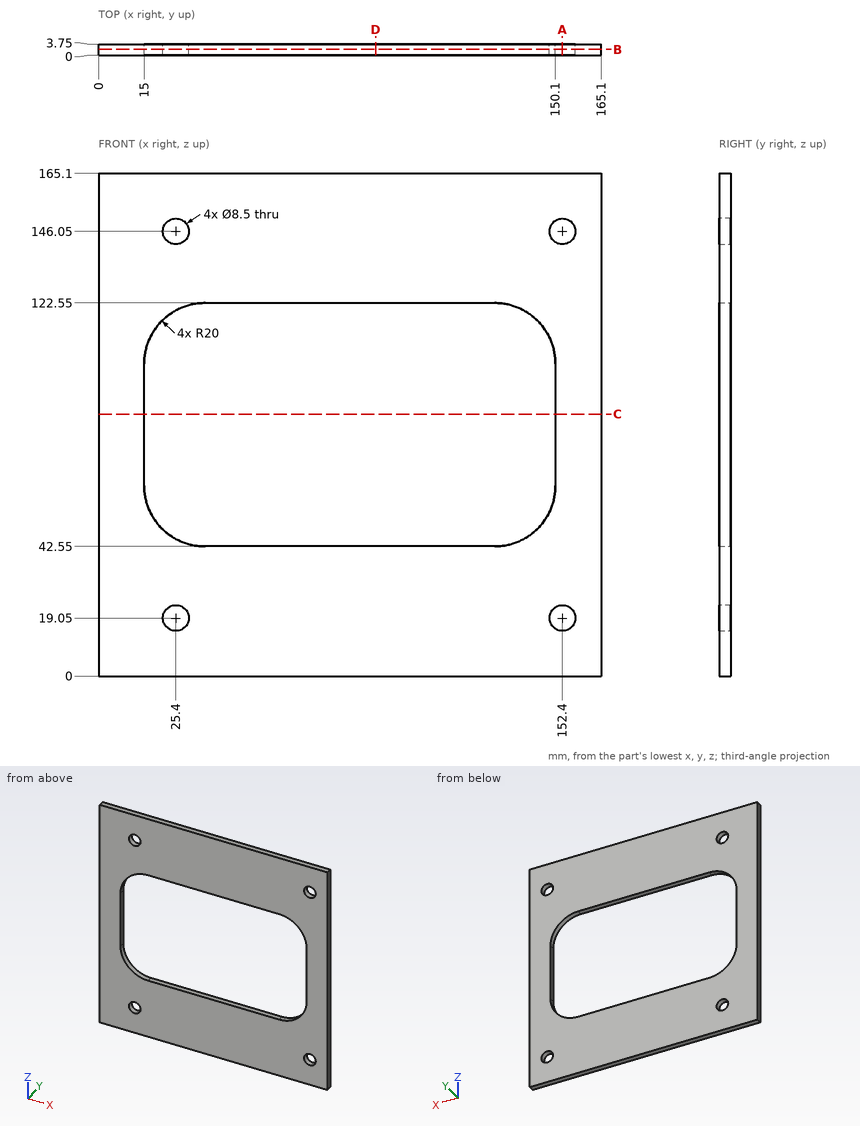
Geometry: see drawing. Coordinates: mm, zero at the bounding-box minimum. Round coordinates to 2 decimals unless told otherwise and drop trailing zeros. Write each loop counter-clockwise with the first axis right and the second up, starting at its lowest first coordinate (ties: lowest second). Pieces come first, ordered by that corner, then holes. Notation, with made-up numbers: M 43,-11.75 L 76,-11.75 A15 cw 76,12.25 Z; hole C -13,-0.5 d4. An arc over 180 degrees is marked long. Answer as a JSON object with one key per item and string values. Group by question number.
(1) Section query A-A on x = 152.4. Output: boundary loops of the cut face in (y, z), then the cut area to 3 significant figures.
(2) Section query C-C on z = 86. Output: boundary loops of the cut face in (x, y).
(3) Ray query, line 1 (Z direction, x = 152.4, y = 2.2); line 2 (X direction, y = 0.9, z = 146.05); line 3 (Z direction, x = 124.5, y = 2.25). Return the intervals inside material, ascending. Write a range as [from, to].
(4) Section query D-D on x = 91. Output: boundary loops of the cut face in (y, z).
(5) Section query B-B on y = 2. Output: boundary loops of the cut face in (x, z), then the cut area to 3 significant figures.
Computed values:
{
 "1": {"outline": "M 0,0 L 3.75,0 L 3.75,14.8 L 0,14.8 Z; M 0,23.3 L 3.75,23.3 L 3.75,141.8 L 0,141.8 Z; M 0,150.3 L 3.75,150.3 L 3.75,165.1 L 0,165.1 Z", "area": "555 mm^2"},
 "2": {"outline": "M 0,0 L 15,0 L 15,3.75 L 0,3.75 Z; M 150.1,0 L 165.1,0 L 165.1,3.75 L 150.1,3.75 Z"},
 "3": {"line 1": "[0, 14.8], [23.3, 141.8], [150.3, 165.1]", "line 2": "[0, 21.15], [29.65, 148.15], [156.65, 165.1]", "line 3": "[0, 42.55], [122.55, 165.1]"},
 "4": {"outline": "M 0,0 L 3.75,0 L 3.75,42.55 L 0,42.55 Z; M 0,122.55 L 3.75,122.55 L 3.75,165.1 L 0,165.1 Z"},
 "5": {"outline": "M 0,0 L 165.1,0 L 165.1,165.1 L 0,165.1 Z; hole M 15,62.55 A20 ccw 35,42.55 L 130.1,42.55 A20 ccw 150.1,62.55 L 150.1,102.55 A20 ccw 130.1,122.55 L 35,122.55 A20 ccw 15,102.55 Z; hole C 25.4,19.05 d8.5; hole C 25.4,146.05 d8.5; hole C 152.4,19.05 d8.5; hole C 152.4,146.05 d8.5", "area": "16,600 mm^2"}
}
